Part model, mm, in its own coordinate system. A direction names the side the tool comes from. Give positions to 0.01 mm unless a question says otherwise; leave off trailing zeros. Write each loop counter-clockwise with the first axis right and the second up, starting at its lowest first coordinate (ties: lowest second). Pieces come first, ordered by that corner, then holes. Notation, with made-up numbers: M 48,78.5 L 103,78.5 A19 ccw 103,101.5 Z; hole C -1.5,-16.5 d3. An arc over 180 degrees is marked long. Use CSV: the item, a comma, the result in double quotes. Start each with the question number.
Item 1: Cut at C-C (z = -64). List the corners of the cut face in (x, y), then the cut area to 3 significant figures.
Item 2: Drill centre lines: line 1 (Y direction, x = 82.55, z = -79.5); line 2 (X direction, y = -3, z = -7.5); line 3 (X direction, y = -9.75, z = -78.5). Where is each one in solid material? Low to high. Write a range as [from, to].
Item 3: Cut at D-D (y = 9.5). List the corners of the cut face in (x, z).
Item 4: Pin check, flat tips, straight feed: pin 1 (12.5 mm diameter, centred on x = 90.5, y = 1, fed in from +Z); pin 2 (4 mm diameter, centred on y = 0, z = -3.5, fed in from -X); pin 3 (12.5 mm diameter, centred on y = -2, z = -39, fed in from +X). Stop position of each tip, or through.
Item 5: Which spindle directions (+Z, -Z, +X, -X, +Y, -Y) get a long thin tool onto all of the face, cutting with end or side? Do faces 1 (the flat face through (63.5, 0, -34)), 2 (the flat face through (-1, 0, 0)), 3 (the flat face through (-79, -6, -76.2)). Say none if no direction does.
Item 6: Cut at A-A (x = -82.55). List the corners of the cut face in (y, z), then the cut area to 3 significant figures.
Item 7: Cut at B-B (y = 0). List the corners of the cut face in (x, z).
from build123d import *

# Parameters (mm, degrees)
F0_W      = 127
F0_H      = 25.4
F1_DEPTH  = 12.7
F2_W      = 12.7
F2_H      = 25.4
F3_DEPTH  = 76.2
F4_W      = 12.7
F4_H      = 25.4
F5_DEPTH  = 76.2
F6_W      = 50.8
F6_H      = 25.4
F7_DEPTH  = 12.7
F8_W      = 50.8
F8_H      = 25.4
F9_DEPTH  = 12.7
F11_DEPTH = 25.4
F13_DEPTH = 25.4
F14_R     = 5.08
F15_R     = 5.08


with BuildPart() as f1:
    # F0 (on Top) → F1 (new body)
    with BuildSketch(Plane.XY):
        Rectangle(F0_W, F0_H)
    extrude(amount=F1_DEPTH)

    # F2 (on face) → F3 (join)
    with BuildSketch(Plane(origin=(0, 0, 0), x_dir=(1, 0, 0), z_dir=(0, 0, -1))):
        with Locations((57.15, 0)):
            Rectangle(F2_W, F2_H)
    extrude(amount=F3_DEPTH)

    # F4 (on face) → F5 (join)
    with BuildSketch(Plane(origin=(0, 0, 0), x_dir=(1, 0, 0), z_dir=(0, 0, -1))):
        with Locations((-57.15, 0)):
            Rectangle(F4_W, F4_H)
    extrude(amount=F5_DEPTH)

    # F6 (on face) → F7 (join)
    with BuildSketch(Plane(origin=(0, 0, -76.2), x_dir=(1, 0, 0), z_dir=(0, 0, -1))):
        with Locations((-76.2, 0)):
            Rectangle(F6_W, F6_H)
    extrude(amount=F7_DEPTH)

    # F8 (on face) → F9 (join)
    with BuildSketch(Plane(origin=(0, 0, -76.2), x_dir=(1, 0, 0), z_dir=(0, 0, -1))):
        with Locations((76.2, 0)):
            Rectangle(F8_W, F8_H)
    extrude(amount=F9_DEPTH)

    # F10 (on face) → F11 (cut)
    with BuildSketch(Plane.XY.offset(-76.2)):
        with BuildLine():
            ThreePointArc((76.2, 0), (82.55, -6.35), (88.9, 0))
            Line((88.9, 0), (76.2, 0))
        make_face()
        with BuildLine():
            Line((76.2, 0), (88.9, 0))
            ThreePointArc((88.9, 0), (82.55, 6.35), (76.2, 0))
        make_face()
    extrude(amount=-F11_DEPTH, mode=Mode.SUBTRACT)

    # F12 (on face) → F13 (cut)
    with BuildSketch(Plane.XY.offset(-76.2)):
        with BuildLine():
            ThreePointArc((-76.2, 0), (-82.55, 6.35), (-88.9, 0))
            Line((-88.9, 0), (-76.2, 0))
        make_face()
        with BuildLine():
            Line((-76.2, 0), (-88.9, 0))
            ThreePointArc((-88.9, 0), (-82.55, -6.35), (-76.2, 0))
        make_face()
    extrude(amount=-F13_DEPTH, mode=Mode.SUBTRACT)

    # F14
    f14_edges = [f1.edges().sort_by_distance(p)[0] for p in [
        (63.5, 0, 12.7),
    ]]
    fillet(f14_edges, radius=F14_R)

    # F15
    f15_edges = [f1.edges().sort_by_distance(p)[0] for p in [
        (-63.5, 0, 12.7),
    ]]
    fillet(f15_edges, radius=F15_R)


solid = f1.part
Worked answers:
1,outline,"M -63.5,-12.7 L -50.8,-12.7 L -50.8,12.7 L -63.5,12.7 Z; M 50.8,-12.7 L 63.5,-12.7 L 63.5,12.7 L 50.8,12.7 Z"
1,area,"645 mm^2"
2,line 1,"y = [-12.7, -6.35], [6.35, 12.7]"
2,line 2,"x = [-63.5, -50.8], [50.8, 63.5]"
2,line 3,"x = [-101.6, -50.8], [50.8, 101.6]"
3,outline,"M -101.6,-88.9 L -50.8,-88.9 L -50.8,0 L 50.8,0 L 50.8,-88.9 L 101.6,-88.9 L 101.6,-76.2 L 63.5,-76.2 L 63.5,7.62 A5.08 ccw 58.42,12.7 L -58.42,12.7 A5.08 ccw -63.5,7.62 L -63.5,-76.2 L -101.6,-76.2 Z"
4,pin 1,"stops at z = -76.2"
4,pin 2,"stops at x = -63.5"
4,pin 3,"stops at x = 63.5"
5,face 1,"+Z, +X, +Y, -Y"
5,face 2,"-Z, +Y, -Y"
5,face 3,"+Z, -X, +Y, -Y"
6,outline,"M -12.7,-88.9 L -6.35,-88.9 L -6.35,-76.2 L -12.7,-76.2 Z; M 6.35,-88.9 L 12.7,-88.9 L 12.7,-76.2 L 6.35,-76.2 Z"
6,area,"161 mm^2"
7,outline,"M -101.6,-88.9 L -88.9,-88.9 L -88.9,-76.2 L -101.6,-76.2 Z; M -76.2,-88.9 L -50.8,-88.9 L -50.8,0 L 50.8,0 L 50.8,-88.9 L 76.2,-88.9 L 76.2,-76.2 L 63.5,-76.2 L 63.5,7.62 A5.08 ccw 58.42,12.7 L -58.42,12.7 A5.08 ccw -63.5,7.62 L -63.5,-76.2 L -76.2,-76.2 Z; M 88.9,-88.9 L 101.6,-88.9 L 101.6,-76.2 L 88.9,-76.2 Z"
